from build123d import *
from OCP.BRepFilletAPI import BRepFilletAPI_MakeChamfer

# Parameters (mm, degrees)
BOSS_EXTRUDE1_DEPTH             = 2
BOSS_EXTRUDE2_REACH             = 41.677
SKETCH2_W                       = 18.358473432
SKETCH2_H                       = 6
BOSS_EXTRUDE2_DIRECTION_2_DEPTH = 10
CUT_EXTRUDE1_DEPTH              = 8
CUT_EXTRUDE2_DEPTH              = 39.833672901
CUT_EXTRUDE2_DEPTH_BACK         = 39.833672901
SKETCH4_W                       = 8
SKETCH4_H                       = 2
CHAMFER1_SIZE                   = 2
CHAMFER2_SIZE                   = 10
CHAMFER2_SIZE2                  = 5.773502692
FILLET1_START                   = -2
FILLET1_DEPTH                   = 5
FILLET1_2_DEPTH                 = 4
BOSS_EXTRUDE3_START             = -6
SKETCH5_W                       = 10
SKETCH5_H                       = 1.6
BOSS_EXTRUDE3_DEPTH             = 10.5


with BuildPart() as part:
    # Sketch1 → Boss-Extrude1 (new, symmetric)
    with BuildSketch(Plane(origin=(0, 0, 0), x_dir=(1, 0, 0), z_dir=(0, 1, 0))):
        Polygon((-8, 0), (0, 0), (0, -1.2), (-9.179236716, -1.2), (-9.402843228, 11.610408514), (-12.023292949, 15.352798559), (-21.634559182, 32), (-20.248918536, 32), (-11.01025903, 15.998172342), (-8.209428877, 11.998172342), align=None)
    boss_extrude1 = extrude(amount=BOSS_EXTRUDE1_DEPTH, both=True)

    # Mirror1: Boss-Extrude1 across plane
    add(boss_extrude1.mirror(Plane(origin=(0, 2, 0), x_dir=(0, 0, 1), z_dir=(-1, 0, 0))))

    # Boss-Extrude2: up to this face of the body (flat: up to its plane)
    boss_extrude2_end = Plane(part.part.faces().sort_by_distance((0, 0, 0))[0])
    # Sketch2 → Boss-Extrude2 (add, up to the picked face)
    with BuildSketch(Plane.XY.offset(1.2), mode=Mode.PRIVATE) as boss_extrude2_sk1:
        with Locations((0, -1)):
            Rectangle(SKETCH2_W, SKETCH2_H)
    boss_extrude2_tool1 = split(extrude(boss_extrude2_sk1.sketch, amount=-BOSS_EXTRUDE2_REACH, mode=Mode.PRIVATE), bisect_by=boss_extrude2_end, keep=Keep.BOTH, mode=Mode.PRIVATE)
    add(boss_extrude2_tool1.solids().sort_by(Axis((0, -1, 1.2), (0, 0, -1)))[0])

    # Sketch2 → Boss-Extrude2 direction 2 (add)
    with BuildSketch(Plane.XY.offset(1.2)):
        with Locations((0, -1)):
            Rectangle(SKETCH2_W, SKETCH2_H)
    extrude(amount=BOSS_EXTRUDE2_DIRECTION_2_DEPTH)

    # Sketch3 → Cut-Extrude1 (cut)
    with BuildSketch(Plane.XY.offset(11.2)):
        with BuildLine():
            Line((-1.5, 1.826658805), (-1.5, 2))
            Line((-1.5, 2), (1.5, 2))
            Line((1.5, 2), (1.5, 1.826658805))
            ThreePointArc((1.5, 1.826658805), (3.2, -1), (1.5, -3.826658805))
            Line((1.5, -3.826658805), (1.5, -4))
            Line((1.5, -4), (-1.5, -4))
            Line((-1.5, -4), (-1.5, -3.826658805))
            ThreePointArc((-1.5, -3.826658805), (-3.2, -1), (-1.5, 1.826658805))
        make_face()
    extrude(amount=-CUT_EXTRUDE1_DEPTH, mode=Mode.SUBTRACT)

    # Sketch4 → Cut-Extrude2 (cut, two sides: drawn at the far end of the back side and taken through both)
    with BuildSketch(Plane(origin=(0, 0, 0), x_dir=(1, 0, 0), z_dir=(0, 1, 0)).offset(-CUT_EXTRUDE2_DEPTH_BACK)):
        with Locations((0, -4.2)):
            Rectangle(SKETCH4_W, SKETCH4_H)
    extrude(amount=CUT_EXTRUDE2_DEPTH + CUT_EXTRUDE2_DEPTH_BACK, mode=Mode.SUBTRACT)

    # Chamfer1
    chamfer1_edges = [part.edges().sort_by_distance(p)[0] for p in [
        (8.589618358, -2, 0),
        (-8.589618358, -2, 0),
    ]]
    chamfer(chamfer1_edges, length=CHAMFER1_SIZE - 0.0001)  # a hair under: the kernel refuses the full size

    # Chamfer2: one chamfer whose edges measure the first distance from different faces: ONE call of the kernel's chamfer builder (chamfer() names one face for all edges)
    chamfer2_edges_1 = [part.edges().sort_by_distance(p)[0] for p in [
        (9.179236716, -1, 11.2),
    ]]
    chamfer2_side_1 = [part.faces().sort_by_distance(p)[0] for p in [
        (9.179236716, -1.126288177, 5.77807488),
    ]]
    chamfer2_edges_2 = [part.edges().sort_by_distance(p)[0] for p in [
        (-9.179236716, -1, 11.2),
    ]]
    chamfer2_side_2 = [part.faces().sort_by_distance(p)[0] for p in [
        (-9.179236716, -1.126288177, 5.77807488),
    ]]
    chamfer2 = BRepFilletAPI_MakeChamfer(part.part.solid().wrapped)
    for e in chamfer2_edges_1:
        chamfer2.Add(CHAMFER2_SIZE, CHAMFER2_SIZE2, e.wrapped, chamfer2_side_1[0].wrapped)  # the first distance lies on this face
    for e in chamfer2_edges_2:
        chamfer2.Add(CHAMFER2_SIZE, CHAMFER2_SIZE2, e.wrapped, chamfer2_side_2[0].wrapped)  # the first distance lies on this face
    add(Compound.cast(chamfer2.Shape()), mode=Mode.REPLACE)

    # Fillet1: read off the stored shape, not the designer's step
    # Fillet1 outline → Fillet1 (cut)
    with BuildSketch(Plane(origin=(0, 0, 0), x_dir=(1, 0, 0), z_dir=(0, 1, 0)).offset(FILLET1_START)):
        with BuildLine():
            Line((12.023292949, 15.352798559), (12.285258606, 15.806536388))
            ThreePointArc((12.285258606, 15.806536388), (12.013651111, 15.358941087), (11.722778292, 14.923619151))
            Line((11.722778292, 14.923619151), (12.023292949, 15.352798559))
        make_face()
        with BuildLine():
            ThreePointArc((8.145400044, 8.329962936), (8.73089419, 11.828737991), (10.313747854, 15.003451295))
            Line((10.313747854, 15.003451295), (8.209428877, 11.998172342))
            Line((8.209428877, 11.998172342), (8.145400044, 8.329962936))
        make_face()
        with BuildLine():
            Line((-12.023292949, 15.352798559), (-11.722778292, 14.923619151))
            ThreePointArc((-11.722778292, 14.923619151), (-12.013651111, 15.358941087), (-12.285258606, 15.806536388))
            Line((-12.285258606, 15.806536388), (-12.023292949, 15.352798559))
        make_face()
        with BuildLine():
            Line((-8.209428877, 11.998172342), (-10.313747854, 15.003451295))
            ThreePointArc((-10.313747854, 15.003451295), (-8.73089419, 11.828737991), (-8.145400044, 8.329962936))
            Line((-8.145400044, 8.329962936), (-8.209428877, 11.998172342))
        make_face()
    extrude(amount=FILLET1_DEPTH, mode=Mode.SUBTRACT)

    # Fillet1 2 outline → Fillet1 2 (add)
    with BuildSketch(Plane(origin=(0, 0, 0), x_dir=(1, 0, 0), z_dir=(0, 1, 0)).offset(FILLET1_START)):
        with BuildLine():
            ThreePointArc((9.338814395, 7.942199107), (9.924308541, 11.440974162), (11.507162205, 14.615687466))
            Line((11.507162205, 14.615687466), (9.402843228, 11.610408514))
            Line((9.402843228, 11.610408514), (9.338814395, 7.942199107))
        make_face()
        with BuildLine():
            ThreePointArc((11.272224688, 16.45191017), (11.000617192, 16.00431487), (10.709744374, 15.568992934))
            Line((10.709744374, 15.568992934), (11.01025903, 15.998172342))
            Line((11.01025903, 15.998172342), (11.272224688, 16.45191017))
        make_face()
        with BuildLine():
            Line((-9.402843228, 11.610408514), (-11.507162205, 14.615687466))
            ThreePointArc((-11.507162205, 14.615687466), (-9.924308541, 11.440974162), (-9.338814395, 7.942199107))
            Line((-9.338814395, 7.942199107), (-9.402843228, 11.610408514))
        make_face()
        with BuildLine():
            ThreePointArc((-10.709744374, 15.568992934), (-11.000617192, 16.00431487), (-11.272224688, 16.45191017))
            Line((-11.272224688, 16.45191017), (-11.01025903, 15.998172342))
            Line((-11.01025903, 15.998172342), (-10.709744374, 15.568992934))
        make_face()
    extrude(amount=FILLET1_2_DEPTH)

    # Sketch5 → Boss-Extrude3 (add)
    with BuildSketch(Plane.XZ.offset(4).offset(BOSS_EXTRUDE3_START)):
        with Locations((0, 0.8)):
            Rectangle(SKETCH5_W, SKETCH5_H)
    extrude(amount=BOSS_EXTRUDE3_DEPTH)


solid = part.part
The listing builds one solid part. Answer for the finished solid, in the listing's coordinates (mm). A direction names the side the tool comes from. Coordinates: 2 decimals unless noted, no trailing zeros. Loops run counter-clockwise (first coordinate to the right, second up) from the corner with the lowest first, then second, coordinate; pieces in that order, holes last. Notation, with made-up numbers: M -33.5,47.25 L 11.5,47.25 A14 ccw 11.5,56.25 Z; hole C 38.25,8 d3. An arc over 180 degrees is marked long. Answer in a Markdown table with one row per item.
1) Given pin 1 (1.6 mm diameter, centred on y = -2, z = 4.5, fed in from +X); pin 2 (0.8 mm diameter, centred on y = -5, z = 1, fed in from +X); pin 3 (15 mm diameter, centred on x = -15, z = -22.5, fed in from -Y); pin 4 (4 mm diameter, centred on x = 15.5, z = -25.5, fed in from +Y), each flat-ended and moving along its own axis, determine where each tip first touches the part or whether it passes through.
Answers below:
| item | result |
|---|---|
| pin 1 | x = 7.74 |
| pin 2 | x = 5 |
| pin 3 | y = -2 |
| pin 4 | y = 2 |
2) Find section D-D (x = 17.5). Determine the outline of the cut face in (y, z).
Answers below:
| item | result |
|---|---|
| outline | M -2,-27.24 L 2,-27.24 L 2,-24.84 L -2,-24.84 Z |
3) Find section C-C (z = 7.5). Determine the outline of the cut face in (x, y).
Answers below:
| item | result |
|---|---|
| outline | M -5.54,-4 L -1.5,-4 L -1.5,-3.83 A3.2 cw -1.5,1.83 L -1.5,2 L -5.54,2 Z; M 1.5,-4 L 5.54,-4 L 5.54,2 L 1.5,2 L 1.5,1.83 A3.2 cw 1.5,-3.83 Z |
4) Find section B-B (y = -4.75). Determine the outline of the cut face in (x, z), then the cut area to 3 significant figures.
Answers below:
| item | result |
|---|---|
| outline | M -5,0 L 5,0 L 5,1.6 L -5,1.6 Z |
| area | 16.0 mm^2 |
5) Find the intervals of material crossed by probe 1 along Z at (x, y) = (0, -2.75); probe 2 along X at (y, z) = (-1.25, -26.5); probe 3 along X at (y, z) = (-0.75, -18), in increasing order.
Answers below:
| item | result |
|---|---|
| probe 1 | 0 to 3.2 |
| probe 2 | -18.46 to -17.07, 17.07 to 18.46 |
| probe 3 | -13.55 to -12.17, 12.17 to 13.55 |
6) Determine the mould class of faces 5 (the flat face through (3.6, -1, 5.2)), 6 (the flat face through (21, 0, -32)), 7 (the flat face through (16.9, 0, -23.8)) for opening direction X: released by +X, released by -X, zero draft, split by the parting line, or undercut.
Answers below:
| item | result |
|---|---|
| face 5 | undercut |
| face 6 | zero draft |
| face 7 | released by +X |
7) Which of the six approach directions +Z, -Z, +X, -X, +Y, -Y give full straight-line access (tool end or side, diameter ignored) to faces 1 (the cylindrical face through (8.716, -0.028, -11.781)), 2 (the flat face through (4, -1, 4)), 3 (the cylindrical face through (-3.2, -1, 8.2)), 4 (the flat face through (0, -6, 1.6))?
Answers below:
| item | result |
|---|---|
| face 1 | -Z, +Y, -Y |
| face 2 | +Y, -Y |
| face 3 | +Z |
| face 4 | +Z, +X, -X, -Y |
8) Find section A-A (z = -26.5). Determine the outline of the cut face in (x, y).
Answers below:
| item | result |
|---|---|
| outline | M -18.46,-2 L -17.07,-2 L -17.07,2 L -18.46,2 Z; M 17.07,-2 L 18.46,-2 L 18.46,2 L 17.07,2 Z |
